Autodesk Inventor part; units mm, degrees
ref_plane "YZ Plane" through (0, 0, 0) normal (1, 0, 0) x (0, 1, 0)
ref_plane "XZ Plane" through (0, 0, 0) normal (0, 1, 0) x (-1, 0, 0)
ref_plane "XY Plane" through (0, 0, 0) normal (0, 0, 1) x (1, 0, 0)
sketch "スケッチ1" plane through (0, 0, 0) normal (1, 0, 0) x (0, 1, 0)
  circle A0 centre (0, 0) radius 4.25
  circle A1 centre (0, 0) radius 6 construction
  circle A2 centre (6, 0) radius 0.8
  line L0 (-14, 0) -> (14, 0)
  circle A3 centre (4.2426, 4.2426) radius 0.8
  circle A4 centre (0, 6) radius 0.8
  circle A5 centre (-4.2426, 4.2426) radius 0.8
  circle A6 centre (-6, 0) radius 0.8
  circle A7 centre (-4.2426, -4.2426) radius 0.8
  circle A8 centre (0, -6) radius 0.8
  circle A9 centre (4.2426, -4.2426) radius 0.8
  circle A10 centre (0, 0) radius 2.4
  line L1 (0, 0) -> (0, 6)
  line L2 (0, 0) -> (2.2961, -5.5433)
  circle A11 centre (0, 0) radius 10
  line L3 (2.2961, -5.5433) -> (3.8268, -9.2388)
  line L4 (0, -9.2388) -> (-10, -9.2388)
  line L5 (-10, -9.2388) -> (-10, 20)
  line L6 (-10, 20) -> (0, 20)
  line L7 (0, 20) -> (0, -9.2388)
  line L8 (0, -6) -> (4.2426, -4.2426) construction
  line L9 (0, -9.2388) -> (3.8268, -9.2388)
  circle A12 centre (0, 6) radius 2.5
  point P0 (0, 5.2)
  point P1 (0, 6.8)
  point P2 (-10, 0)
  point P3 (2.1213, -5.1213)
  point P4 (0, 2.4)
  point P5 (0.9184, -2.2173)
  point P6 (1.4789, 3.9844)
  point P7 (0, 8.5)
  point P8 (1.6264, -3.9265)
  dimension "d0" = 8.5
  dimension "d1" = 12
  dimension "d2" = 1.6
  dimension "d5" = 360
  dimension "d7" = 4.8
  dimension "d8" = 4
  dimension "d21" = 5
  dimension "d23" = 20
extrude "押し出し1" add sketch "スケッチ1" along normal blind 1.5 contours L0 A10 L1 A12 A0 | A0 L2 A10 L0 | L2 L3 L9 L7 A8 A0 | A0 L7 A10 L2 | A10 L2 L0 | L0 L1 A10 | L1 A10 L0 A0 A12 | L7 A8 L4 A11 L0 A6 A0 | A0 L0 A10 L7 | A10 L7 L2 | L7 A10 L0 | L0 A10 L1 | A0 L0 A6 A11 L7 A12 | A11 L4 L9 | A11 L5 L6 L7
sketch "スケッチ3" plane through (1.5, 0, 0) normal (1, 0, 0) x (0, 0, -1)
  circle A0 centre (0, 0) radius 2.5 construction
  line L0 (0, -2.5) -> (-20, -2.5) construction
  line L1 (-20, -2.5) -> (0, -2.5)
  line L2 (0, -2.5) -> (0, -3.5)
  line L3 (0, -3.5) -> (-20, -3.5)
  line L4 (-20, -3.5) -> (-20, -2.5)
  circle A1 centre (0, 0) radius 3.5
  line L5 (-20, 0) -> (-20, -10)
  line L6 (-8.5, 0) -> (-20, 0)
  line L7 (-20, 0) -> (-20, -10)
  line L8 (-20, -10) -> (0, -10)
  arc A2 (0, -10) -> (9.2388, 3.8268) centre (0, 0) ccw
  line L9 (9.2388, 3.8268) -> (3.9265, 1.6264)
  circle A3 centre (4.2426, -4.2426) radius 0.8
  circle A4 centre (-4.2426, -4.2426) radius 0.8
  circle A5 centre (0, -6) radius 0.8
  circle A6 centre (-4.2426, -4.2426) radius 2.5
  circle A7 centre (0, -6) radius 2.5
  circle A8 centre (4.2426, -4.2426) radius 2.5
  circle A9 centre (6, 0) radius 0.8
  circle A10 centre (6, 0) radius 2.5
  arc A11 (-8.5, 0) -> (-3.9844, 1.4789) centre (-6, 0) ccw
  arc A12 (3.9265, 1.6264) -> (-3.9844, 1.4789) centre (0, 0) ccw
  circle A13 centre (0, 0) radius 2.4
  line L10 (3.2336, -1.3394) -> (9.2388, -3.8268)
  line L11 (6, 0) -> (4.2426, -4.2426) construction
  point P0 (6.0349, 2.4998)
  point P1 (6.0349, -2.4998)
  point P2 (2.4998, -6.0349)
  point P3 (-2.4998, -6.0349)
  point P4 (-6.6298, -3.5)
  point P5 (5.1213, -2.1213)
  point P6 (6.0349, -2.4998)
  dimension "d13" = 5
  dimension "d14" = 1
  dimension "d15" = 5
  dimension "d16" = 5
  dimension "d17" = 5
  dimension "d18" = 5
  dimension "d22" = 4.8
extrude "押し出し2" add sketch "スケッチ3" along normal blind 2.5 contours L3 A6 A7 A8 L10 A2 L8 L5 | A13
sketch "スケッチ4" plane through (0, 0, 0) normal (-1, 0, 0) x (0, 0, 1)
  line L0 (3.7223, -10.4472) -> (3.446, -9.9687)
  arc A0 (3.446, -9.9687) -> (0.6267, -8.4769) centre (0.848, -11.4687) ccw
  arc A1 (-1.1087, -8.4274) -> (0.6267, -8.4769) centre (0, 0) ccw
  arc A2 (-1.1087, -8.4274) -> (-4.5, -11.4018) centre (-1.5, -11.4018) ccw
  line L1 (-4.5, -11.4018) -> (-4.5, -11.9059)
  arc A3 (-4.5, -11.9059) -> (-1.875, -14.8824) centre (-1.5, -11.9059) ccw
  arc A4 (-1.875, -14.8824) -> (1.4053, -14.934) centre (0, 0) ccw
  arc A5 (1.4053, -14.934) -> (3.7223, -10.4472) centre (1.1242, -11.9472) ccw
  arc A6 (-8.5, -16) -> (-5.5, -19) centre (-5.5, -16) ccw
  line L2 (-8.5, -16) -> (-8.5, 0)
  arc A7 (8.2057, 2.2174) -> (-8.5, 0) centre (0, 0) ccw
  arc A8 (8.2057, 2.2174) -> (11.1018, 0) centre (11.1018, 3) ccw
  line L3 (11.1018, 0) -> (16, 0)
  arc A9 (19, -3) -> (16, 0) centre (16, -3) ccw
  line L4 (19, -3) -> (19, -16)
  arc A10 (16, -19) -> (19, -16) centre (16, -16) ccw
  line L5 (16, -19) -> (-5.5, -19)
  circle A11 centre (-6, 0) radius 1
  circle A12 centre (-4.2426, 4.2426) radius 1
  circle A13 centre (0, 6) radius 1
  circle A14 centre (4.2426, 4.2426) radius 1
  circle A15 centre (13.8033, -13.8033) radius 0.8
  circle A16 centre (-2.5, -17) radius 0.8
  circle A17 centre (17, -17) radius 0.8
  circle A18 centre (6, 0) radius 1
  circle A19 centre (4.2426, -4.2426) radius 1
  circle A20 centre (-4.2426, -4.2426) radius 1
  circle A21 centre (0, -6) radius 1
  circle A22 centre (0, 0) radius 4.25
  circle A23 centre (17, -3.5) radius 0.8
  arc A24 (12.1835, -8.75) -> (9.7468, -4) centre (9.7468, -7) ccw
  line L6 (9.7468, -4) -> (9.1241, -4)
  arc A25 (9.1241, -4) -> (6.7439, -5.1739) centre (9.1241, -7) ccw
  arc A26 (6.7439, -5.1739) -> (6.878, -7.913) centre (9.4761, -6.413) ccw
  line L7 (6.878, -7.913) -> (7.1869, -8.448)
  arc A27 (7.1869, -8.448) -> (12.1835, -8.75) centre (9.785, -6.948) ccw
  circle A28 centre (-6, 0) radius 0.8
  circle A29 centre (-4.2426, -4.2426) radius 0.8
  circle A30 centre (4.2426, -4.2426) radius 0.8
  circle A31 centre (0, -6) radius 0.8
  arc A32 (3.9844, 1.4789) -> (8.5, 0) centre (6, 0) ccw
  arc A33 (3.9844, 1.4789) -> (-3.9265, 1.6264) centre (0, 0) ccw
  line L8 (-9.2388, 3.8268) -> (-3.9265, 1.6264)
  arc A34 (-9.2388, 3.8268) -> (0, -10) centre (0, 0) ccw
  line L9 (20, -10) -> (0, -10)
  line L10 (20, 0) -> (20, -10)
  line L11 (8.5, 0) -> (20, 0)
  line L12 (12.7468, -10) -> (12.7468, -6.471)
  line L13 (6.4797, -10) -> (6.4797, -6.5597)
  point P0 (-3.6504, -9.3099)
  point P1 (3.4641, -10)
  point P2 (19, -10)
  point P3 (-8.5, -5.2678)
  point P4 (-7.853, 3.2528)
  point P5 (12.7468, -7)
extrude "押し出し3" cut sketch "スケッチ4" against normal through all contours L9 A34 A2 A1 A0 L0 | L13 A26 L7 A27 A24 L12 L9 | A26 A25 L6 A24 A27 L7 | L4 A9 L11 L10 L9 | A34 L8 A7 L2 | A23
sketch "スケッチ5" plane through (4, 0, 0) normal (1, 0, 0) x (0, 0, -1)
  circle A0 centre (-17, -3.5) radius 2.5
  arc A1 (-16.2, -3.5) -> (-17.8, -3.5) centre (-17, -3.5) ccw
  point P0 (0, 0)
  dimension "d26" = 5
extrude "押し出し4" cut sketch "スケッチ5" against normal up to surface (2.5 mm away)
sketch "スケッチ6" plane through (4, 0, 0) normal (1, 0, 0) x (0, 0, -1)
  circle A0 centre (-16, -7) radius 0.8
  circle A1 centre (0, 0) radius 0.8
  point P0 (0, 0)
extrude "押し出し5" cut sketch "スケッチ6" against normal through all
fillet "フィレット1" radius 2 6 edges at (2, -10, 19) (2, -10, 12.7468) (2, -10, 6.4797) (0.75, 3.2528, -7.853) (0.75, 0, 8.5) (0.75, 1.4789, 3.9844)
properties part number "toe_springjoint_bace_under_left"
Work out the finished part from the listing and answer in its coordinate system (mm). A direction names the side the tool comes from. Round coordinates to 2 decimals unless told otherwise and drop trailing zeros. Order: outer loops, then holes, each group sorted by start corner. A loop starts at its lowest first (then second) coordinate and runs counter-clockwise, first axis right, second up. Notation, with made-up numbers: M 51,59.25 L 90,59.25 A28 cw 90,86.25 Z; hole C 34,-15 d5. An arc over 180 degrees is marked long. Put each result on its own line as item: value. Start each with the question number.
Q1. Section A-A, the plane x = 2.5 is taken. Give the number of separate pieces and of enclosed holes in the cut face, and give its area (3 significant figures).
Q2. Flat-ended cylindrical pins translate along their axes: pin 1 (1.1 mm diameter, centred on x = 3, y = -7.5, fed in from -Z); pin 2 (1.5 mm diameter, centred on y = -1.5, z = 7.5, fed in from -X); pin 3 (1 mm diameter, centred on x = 2.5, z = 12.5, fed in from +Y); pin 4 (1.6 mm diameter, centred on x = 1, z = 14.5, fed in from +Y). Find the tip coordinate at first contact, or state that the pin passes through.
Q3. A tool of negligible diameter and unlimited length cuts with its end or side. For faces 1 (the cylindrical face through (0.76, 2.21, -7.55)), 2 (the cylindrical face through (2.732, -6.397, 5.511)), 3 (the flat face through (2, -6, 19)), 4 (the flat face through (2, -7.5, 12.747)), 5 (the flat face through (1, 0, 13)), from which of +Z, -Z, +X, -X, +Y, -Y can it reach the whole face along a straight path? Write none if from no direction.
Q4. For a pull along Z with two mould halves and no side action, classify faces 6 (the flat face through (2, -10, 4)), 7 (the cylindrical face through (2.03, -0.49, 0.63)), 8 (the cylindrical face through (0.74, -0.9, 18.14)), 9 (the cylindrical face through (2.732, -2.024, -1.29)) as pulls with the +Z half, pulls with the -Z half, needs draft (parallel to the pull), parting line crosses it, or undercut.
Q5. Section D-D, the plane z = 7.5 is taken. Write down the section's boundary in (x, y).
Q6. Section C-C, the plane y = 0.25 is taken. Write down the section's boundary in (x, z), and give its area (3 significant figures).
Q7. Straight lines are drawn through the part: L1, parallel to Z at x = 0.8, y = -0.5; L2, parallel to Z at x = 0.85, y = -6; L3, parallel to Z at x = 1.95, y = -8. For each, find the intervals that lie inside material, in ascending order. Write a range as [from, to].
Findings below:
1. separate pieces: 2
1. enclosed holes: 2
1. area: 80.8 mm^2
2. pin 1: stops at z = -7.19
2. pin 2: stops at x = 0
2. pin 3: stops at y = -3.5
2. pin 4: stops at y = 0
3. face 1: +X, -X, +Y
3. face 2: +X
3. face 3: +Z, +X, -X, +Y, -Y
3. face 4: +X, -X, -Y
3. face 5: +Z, +X, -X, +Y
4. face 6: needs draft
4. face 7: undercut
4. face 8: pulls with the +Z half
4. face 9: parting line crosses it
5. outline: M 0,-4.48 L 4,-4.48 L 4,-3.5 L 1.5,-3.5 L 1.5,-2 L 0,-2 Z
6. outline: M 0,-8.5 L 1.5,-8.5 L 1.5,-6.76 L 0,-6.76 Z; M 0,-5.24 L 1.5,-5.24 L 1.5,-2.39 L 4,-2.39 L 4,-0.76 L 0,-0.76 Z; M 0,0.76 L 4,0.76 L 4,2.39 L 1.5,2.39 L 1.5,3.51 L 0,3.51 Z
6. area: 21.6 mm^2
7. L1: z = [-8.5, -6.62], [-5.38, -0.62], [0.62, 3.55], [8.71, 17.66]
7. L2: z = [-8, -0.8], [0.8, 6.5], [12.58, 19]
7. L3: z = [-6, -1.5], [1.5, 6.48], [12.75, 19]
